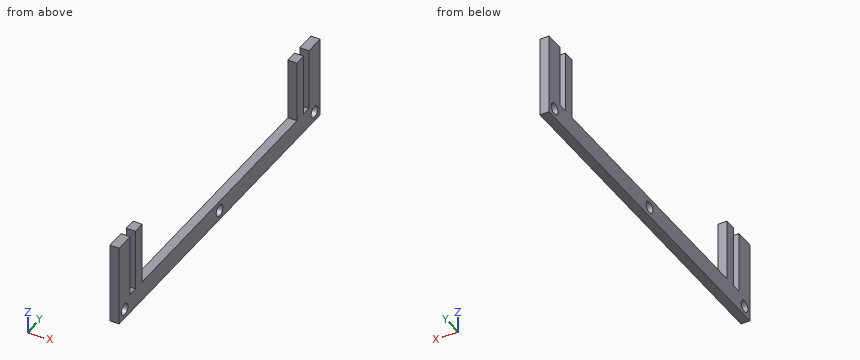
```python
from build123d import *

# Parameters (mm, degrees)
SKETCH1_W           = 114.3
SKETCH1_H           = 26.643356644
BOSS_EXTRUDE1_DEPTH = 2.9718
SKETCH2_W           = 2.9718
SKETCH2_H           = 20.293356644
SKETCH2_W_2         = 88.0364
CUT_EXTRUDE1_DEPTH  = 3.175
SKETCH3_R           = 1.905
CUT_EXTRUDE2_DEPTH  = 3.175


with BuildPart() as part:
    # Sketch1 → Boss-Extrude1 (new body)
    with BuildSketch(Plane.YZ):
        Rectangle(SKETCH1_W, SKETCH1_H)
    extrude(amount=BOSS_EXTRUDE1_DEPTH)

    # Sketch2 → Cut-Extrude1 (cut)
    with BuildSketch(Plane.YZ.offset(2.9718)):
        with Locations((-49.3141, 3.175)):
            Rectangle(SKETCH2_W, SKETCH2_H)
        with Locations((49.3141, 3.175)):
            Rectangle(SKETCH2_W, SKETCH2_H)
        with Locations((0, 3.175)):
            Rectangle(SKETCH2_W_2, SKETCH2_H)
    extrude(amount=-CUT_EXTRUDE1_DEPTH, mode=Mode.SUBTRACT)

    # Sketch3 → Cut-Extrude2 (cut)
    with BuildSketch(Plane.YZ.offset(2.9718)):
        with Locations(Location((0, -10.209266023, 0), (0, 0, 270))):
            Circle(SKETCH3_R)
        with Locations(Location((-53.975, -10.209266023, 0), (0, 0, 270))):
            Circle(SKETCH3_R)
        with Locations(Location((53.975, -10.209266023, 0), (0, 0, 270))):
            Circle(SKETCH3_R)
    extrude(amount=-CUT_EXTRUDE2_DEPTH, mode=Mode.SUBTRACT)


solid = part.part
```
Read the model definition and answer for the solid it produces. Units are mm, in the model's axes. Round coordinates to 2 decimals unless told otherwise and drop trailing zeros. Write each loop counter-clockwise with the first axis right and the second up, starting at its lowest first coordinate (ties: lowest second). Pieces come first, ordered by that corner, then holes. Notation, with made-up numbers: M 51.25,83.25 L 73.25,83.25 A27 ccw 73.25,112.25 Z; hole C -37.75,-12 d2. An arc over 180 degrees is marked long. One line per item, written item: value.
Q1. Find section B-B on y = 0. Write down the section's boundary in (x, z), plus the area to 3 significant figures.
Data:
outline: M 0,-13.32 L 2.97,-13.32 L 2.97,-12.11 L 0,-12.11 Z; M 0,-8.3 L 2.97,-8.3 L 2.97,-6.97 L 0,-6.97 Z
area: 7.55 mm2
Q2. Find section A-A on z = -5.5. Write down the section's boundary in (x, y), plus the area to 3 significant figures.
Data:
outline: M 0,-57.15 L 2.97,-57.15 L 2.97,-50.8 L 0,-50.8 Z; M 0,-47.83 L 2.97,-47.83 L 2.97,-44.02 L 0,-44.02 Z; M 0,44.02 L 2.97,44.02 L 2.97,47.83 L 0,47.83 Z; M 0,50.8 L 2.97,50.8 L 2.97,57.15 L 0,57.15 Z
area: 60.4 mm2
Q3. A flat-ended cylindrical pin translates along its axis: pin 1 Ø1.5 at (x, y) = (1, -49) entering from +Z. Find the tip coordinate at first contact, or state that the pin passes through.
Data:
pin 1: z = -6.97
Q4. Find section C-C on x = 1.4. Write down the section's boundary in (y, z) (3 decimals), plus the area to 3 significant figures.
Data:
outline: M -57.15,-13.322 L 57.15,-13.322 L 57.15,13.322 L 50.8,13.322 L 50.8,-6.972 L 47.828,-6.972 L 47.828,13.322 L 44.018,13.322 L 44.018,-6.972 L -44.018,-6.972 L -44.018,13.322 L -47.828,13.322 L -47.828,-6.972 L -50.8,-6.972 L -50.8,13.322 L -57.15,13.322 Z; hole C -53.975,-10.209 d3.81; hole C 0,-10.209 d3.81; hole C 53.975,-10.209 d3.81
area: 1,100 mm2
Q5. Straight lines are drawn through the part: line 1 (Y direction, x = 1.9, z = -10.5); line 2 (Y direction, x = 0.35, z = 12.25); line 3 (Z direction, x = 2.5, y = 5.5). For each, find the intervals that lie inside material, in ascending order. Write a range as [from, to].
Data:
line 1: [-57.15, -55.86], [-52.09, -1.88], [1.88, 52.09], [55.86, 57.15]
line 2: [-57.15, -50.8], [-47.83, -44.02], [44.02, 47.83], [50.8, 57.15]
line 3: [-13.32, -6.97]
